Part print with two shaded views. Sizes in mm from the minimum x, y, z corner. A direction names the side the tool comes from. Coordinates: 2 decimals unless noted, no trailing zeros. Order: outer loops, then holes, each group sorted by start corner. A loop starts at its lowest first (then second) coordinate and runs counter-clockwise, first axis right, second up. Notation, with made-up numbers: M -26.75,1.25 L -2.75,1.25 A15 cw -2.75,6.25 Z; hole C -18.75,-10 d9. An arc over 180 degrees is marked long. Answer in a Markdown table with one row per item. Add a question column.
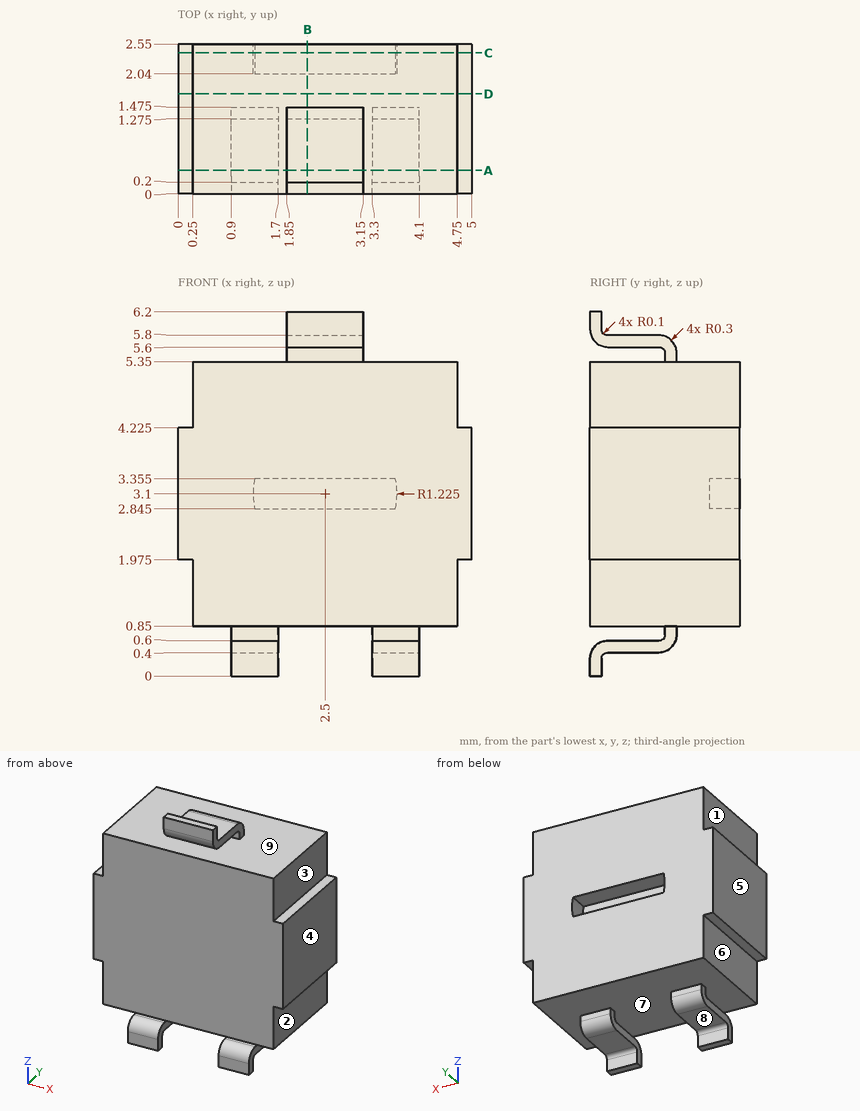
(1) Drop flat-ended pins along their axis: P1, Ø0.9, axis at y = 0.5, z = 6, coming from the +X side; P2, Ø0.7, axis at y = 1, z = 6, coming from the -X side; P3, Ø1, axis at x = 4, y = 0.5, coming from the +Z side. Give the stop position or say it passes through.
(2) 3-axis set-ups, long thin cutter, end or side, ignore diameter. For the marked faces 1, 2, 3, 4 and 5: which of +Z, -Z, +X, -X, +Y, -Y reach the whole face in a straight line?
(3) Slice it at C-C (y = 2.4). List the corners of the cut face in (x, z) (3 decimals), and give its area (3 significant figures).
(4) Wall check: line 1 (Z direction, x = 1.3, y = 1.15); line 2 (Z direction, x = 2.25, y = 0.5); line 3 (Z direction, x = 1.8, y = 1.65). Give the ranges that are in metal, low to high.
(5) Slice it at B-B (x = 2.2). List the corners of the cut face in (y, z) (3 decimals), and give its area (3 significant figures).
(6) Slice it at A-A (y = 0.4). List the corners of the cut face in (x, z) (3 decimals), and give its area (3 significant figures).
(7) Pull direction Z, two halves, no side cores. Call the marked faces 6, 7, 8 and 9: pulls with the +Z half, pulls with the -Z half, needs draft (parallel to the pull), parting line crosses it, or undercut.
(8) Slice it at D-D (y = 1.7). List the corners of the cut face in (x, z) (3 decimals).
Computed:
| question | item | result |
|---|---|---|
| 1 | P1 | stops at x = 3.15 |
| 1 | P2 | stops at x = 1.85 |
| 1 | P3 | stops at z = 5.35 |
| 2 | face 1 | +Z, -X, +Y, -Y |
| 2 | face 2 | -Z, +X, +Y, -Y |
| 2 | face 3 | +Z, +X, +Y, -Y |
| 2 | face 4 | +Z, -Z, +X, +Y, -Y |
| 2 | face 5 | +Z, -Z, -X, +Y, -Y |
| 3 | outline | M 0,1.975 L 0.25,1.975 L 0.25,0.85 L 4.75,0.85 L 4.75,1.975 L 5,1.975 L 5,4.225 L 4.75,4.225 L 4.75,5.35 L 0.25,5.35 L 0.25,4.225 L 0,4.225 Z; hole M 1.302,2.845 L 3.698,2.845 A1.225 ccw 3.698,3.355 L 1.302,3.355 A1.225 ccw Z |
| 3 | area | 20.1 mm^2 |
| 4 | line 1 | z = 0.4 to 0.6, 0.85 to 5.35 |
| 4 | line 2 | z = 0.85 to 5.35, 5.6 to 5.8 |
| 4 | line 3 | z = 0.85 to 5.35 |
| 5 | outline | M 0,0.85 L 2.55,0.85 L 2.55,2.845 L 2.04,2.845 L 2.04,3.355 L 2.55,3.355 L 2.55,5.35 L 1.475,5.35 L 1.475,5.5 A0.3 ccw 1.175,5.8 L 0.3,5.8 A0.1 cw 0.2,5.9 L 0.2,6.2 L 0,6.2 L 0,5.9 A0.3 ccw 0.3,5.6 L 1.175,5.6 A0.1 cw 1.275,5.5 L 1.275,5.35 L 0,5.35 Z |
| 5 | area | 11.6 mm^2 |
| 6 | outline | M 0,1.975 L 0.25,1.975 L 0.25,0.85 L 4.75,0.85 L 4.75,1.975 L 5,1.975 L 5,4.225 L 4.75,4.225 L 4.75,5.35 L 0.25,5.35 L 0.25,4.225 L 0,4.225 Z; M 0.9,0.4 L 1.7,0.4 L 1.7,0.6 L 0.9,0.6 Z; M 1.85,5.6 L 3.15,5.6 L 3.15,5.8 L 1.85,5.8 Z; M 3.3,0.4 L 4.1,0.4 L 4.1,0.6 L 3.3,0.6 Z |
| 6 | area | 22.0 mm^2 |
| 7 | face 6 | needs draft |
| 7 | face 7 | undercut |
| 7 | face 8 | pulls with the -Z half |
| 7 | face 9 | undercut |
| 8 | outline | M 0,1.975 L 0.25,1.975 L 0.25,0.85 L 4.75,0.85 L 4.75,1.975 L 5,1.975 L 5,4.225 L 4.75,4.225 L 4.75,5.35 L 0.25,5.35 L 0.25,4.225 L 0,4.225 Z |
